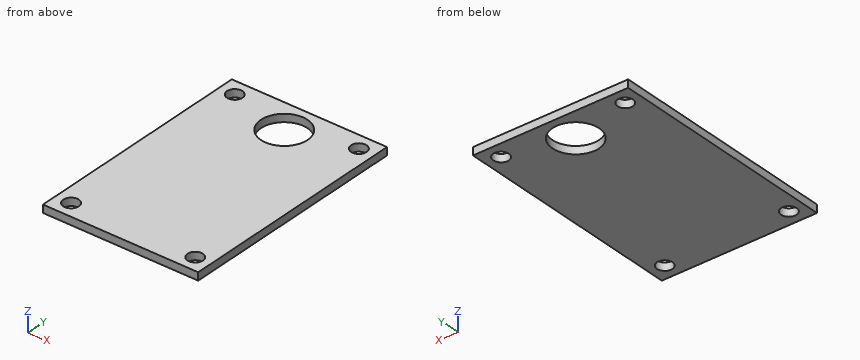
Autodesk Fusion 360 part; units mm, degrees
sketch "Sketch1" plane through (0, 0, 0) normal (0, 0, 1) x (1, 0, 0)
  line L0 (0, 0) -> (100, 0)
  line L1 (100, 0) -> (100, -150)
  line L2 (0, 0) -> (0, -150)
  line L3 (0, -150) -> (100, -150)
  dimension "d1" = 100
  dimension "d2" = 150
extrude "Extrude1" add sketch "Sketch1" along normal blind 5
hole "Hole1" at (10, -10, 5) direction (0, 0, -1) diameter 10 depth 5 tip angle 180
hole "Hole2" at (90, -10, 5) direction (0, 0, -1) diameter 10 depth 5 tip angle 180
hole "Hole3" at (10, -140, 5) direction (0, 0, -1) diameter 10 depth 5 tip angle 180
hole "Hole4" at (90, -140, 5) direction (0, 0, -1) diameter 10 depth 5 tip angle 180
hole "Hole5" at (50, -20, 5) direction (0, 0, -1) diameter 30 depth 5 tip angle 180
Check sheet for the modelled part. Datum: model origin and axes. Units: mm. Round coordinates to 2 decimals unless told otherwise and drop trailing zeros. Order: outer loops, then holes, each group sorted by start corner. A loop starts at its lowest first (then second) coordinate and runs counter-clockwise, first axis right, second up.
1) Section check A-A (x = 50). Record the boundary of the cut face in (y, z), and give its area (3 significant figures).
2) Go/stop test with a flat-tipped pin: pin 1 Ø8 at (x, y) = (10, -140) entering from +Z. Record where the tip stops, or that it passes through.
3) Scan lines: line 1 (Y direction, x = 10, z = 1.4); line 2 (X direction, y = -140, z = 3.75); line 3 (X direction, y = -11, z = 2.95). Record each from-to range of solid material in increasing order.
4) Section check C-C (y = -20). Record the boundary of the cut face in (x, z).
5) Section check B-B (x = 10). Record the boundary of the cut face in (y, z).
6) Section check D-D (z = 2.1). Record the boundary of the cut face in (x, y), and give its area (3 significant figures).
Result:
1. outline: (-150, 0) - (-35, 0) - (-35, 5) - (-150, 5) - close; (-5, 0) - (0, 0) - (0, 5) - (-5, 5) - close
1. area: 600 mm2
2. pin 1: passes through
3. line 1: y = -150 to -145, -135 to -15, -5 to 0
3. line 2: x = 0 to 5, 15 to 85, 95 to 100
3. line 3: x = 0 to 5.1, 14.9 to 38, 62 to 85.1, 94.9 to 100
4. outline: (0, 0) - (35, 0) - (35, 5) - (0, 5) - close; (65, 0) - (100, 0) - (100, 5) - (65, 5) - close
5. outline: (-150, 0) - (-145, 0) - (-145, 5) - (-150, 5) - close; (-135, 0) - (-15, 0) - (-15, 5) - (-135, 5) - close; (-5, 0) - (0, 0) - (0, 5) - (-5, 5) - close
6. outline: (0, -150) - (100, -150) - (100, 0) - (0, 0) - close; hole circle Ø10 at (10, -140); hole circle Ø10 at (10, -10); hole circle Ø30 at (50, -20); hole circle Ø10 at (90, -140); hole circle Ø10 at (90, -10)
6. area: 14,000 mm2
